from build123d import *

# Parameters (mm, degrees)
SKETCH1_R            = 57
EXTRUDE4_DEPTH       = 7.5
EXTRUDE5_DEPTH       = 7.5
EXTRUDE5_DEPTH_BACK  = 5
SKETCH_R             = 60
SKETCH_R_2           = 57
SKETCH2_R            = 6
SKETCH2_R_2          = 14
EXTRUDE6_DEPTH       = 87.168439698
M5_CLEARANCE_HOLE1_D = 5.5
SKETCH6_R            = 14.8
EXTRUDE7_DEPTH       = 2.5
EXTRUDE8_START       = -16.8000001
EXTRUDE8_OUTLINE_R   = 2
EXTRUDE8_DEPTH       = 2.135757978
EXTRUDE8_START_2     = -3
EXTRUDE8_2_DEPTH     = 6


with BuildPart() as part:
    # Sketch1 → Extrude4 (new, symmetric)
    with BuildSketch(Plane(origin=(0, 0, 0), x_dir=(1, 0, 0), z_dir=(0, 1, 0))):
        with Locations(Location((0, 0, 0), (0, 0, 270))):
            Circle(SKETCH1_R)
    extrude(amount=EXTRUDE4_DEPTH, both=True)

    # Sketch → Extrude5 (add, two sides: drawn at the far end of the back side and taken through both)
    with BuildSketch(Plane(origin=(0, 0, 0), x_dir=(1, 0, 0), z_dir=(0, 1, 0)).offset(-EXTRUDE5_DEPTH_BACK)):
        with Locations(Location((0, 0, 0), (0, 0, 270))):
            Circle(SKETCH_R)
        with Locations(Location((0, 0, 0), (0, 0, 270))):
            Circle(SKETCH_R_2, mode=Mode.SUBTRACT)
    extrude(amount=EXTRUDE5_DEPTH + EXTRUDE5_DEPTH_BACK)

    # Sketch2 → Extrude6 (cut, through all)
    with BuildSketch(Plane(origin=(0, 7.5, 0), x_dir=(1, 0, 0), z_dir=(0, 1, 0))):
        with Locations(Location((-37.5, 0, 0), (0, 0, 270))):
            Circle(SKETCH2_R)
        with Locations(Location((37.5, 0, 0), (0, 0, 270))):
            Circle(SKETCH2_R)
        with Locations(Location((0, 0, 0), (0, 0, 270))):
            Circle(SKETCH2_R_2)
    extrude(amount=-EXTRUDE6_DEPTH, mode=Mode.SUBTRACT)

    # M5 Clearance Hole1 (through all)
    with Locations(Plane(origin=(0, 7.5, 0), x_dir=(1, 0, 0), z_dir=(0, 1, 0))):
        with Locations((37.5, 18), (37.5, -18), (-37.5, 18), (-37.5, -18)):
            Hole(M5_CLEARANCE_HOLE1_D / 2)

    # Sketch6 → Extrude7 (cut, symmetric)
    with BuildSketch(Plane(origin=(0, 0, 0), x_dir=(1, 0, 0), z_dir=(0, 1, 0))):
        with Locations(Location((0, 0, 0), (0, 0, 270))):
            Circle(SKETCH6_R)
    extrude(amount=EXTRUDE7_DEPTH, both=True, mode=Mode.SUBTRACT)

    # Extrude8: read off the stored shape, not the designer's step
    # Extrude8 outline → Extrude8 (cut)
    with BuildSketch(Plane.XY.offset(EXTRUDE8_START)):
        Circle(EXTRUDE8_OUTLINE_R)
    extrude(amount=EXTRUDE8_DEPTH, mode=Mode.SUBTRACT)

    # Extrude8 2 outline → Extrude8 2 (add)
    with BuildSketch(Plane(origin=(0, 0, 0), x_dir=(1, 0, 0), z_dir=(0, 1, 0)).offset(EXTRUDE8_START_2)):
        with BuildLine():
            ThreePointArc((-2e-09, 16.8), (1.002059984, 16.770088723), (2.000551768, 16.680461403))
            Line((2.000551768, 16.680461403), (3, 16.56059374))
            Line((3, 16.56059374), (3, 16.8000001))
            Line((3, 16.8000001), (-2e-09, 16.8))
        make_face()
        with BuildLine():
            ThreePointArc((-2.000001192, 16.680527427), (-1.001783219, 16.770105259), (-2e-09, 16.8))
            Line((-2e-09, 16.8), (-3, 16.8000001))
            Line((-3, 16.8000001), (-3, 16.560627213))
            Line((-3, 16.560627213), (-2.000001192, 16.680527427))
        make_face()
    extrude(amount=EXTRUDE8_2_DEPTH)


solid = part.part
For this review, take the finished solid that the model builds, in its own axes (mm). A direction names the side the tool comes from. Give positions to 0.01 mm unless a question says otherwise; leave off trailing zeros. Loops run counter-clockwise (first coordinate to the right, second up) from the corner with the lowest first, then second, coordinate; pieces in that order, holes last. Notation, with made-up numbers: (34.25, -12.5) -> (89.25, -12.5) arc R19 cw to (89.25, -1.5) -> close; hole circle Ø5 at (12.25, 53). An arc over 180 degrees is marked (long way). One line per question, with ' | ' between items.
1) For faces 4 (the cylindrical face through (40.247, -0.105, 17.879)), 5 (the cylindrical face through (-55.645, -6.232, -12.356)), 6 (the cylindrical face through (-5.67, 0.04, 13.67)), list the 3-axis set-ups (+Z, -Z, +X, -X, +Y, -Y) from which the entire face can be reached by the end or side of a thin tool; tool diameter is ignored.
Resolved:
face 4: +Y, -Y | face 5: -Y | face 6: none
2) The part is to be moulded in two halves that separate along X. For faces 1 (the cylindrical face through (2.64, 1.16, -59.94)), 2 (the flat face through (-11, -2.5, -9)), 3 (the flat face through (-22, -5, 53)), say which applies: +X half, -X half, draft (parallel to the pull), parting line (faces both ways), or undercut.
Resolved:
face 1: parting line | face 2: undercut | face 3: draft
3) We need section B-B (z = 3.5). Write out the cut boundary in (x, y).
Resolved:
outline: (-59.9, -5) -> (-56.89, -5) -> (-56.89, -7.5) -> (-42.37, -7.5) -> (-42.37, 7.5) -> (-59.9, 7.5) -> close; (-32.63, -7.5) -> (-13.56, -7.5) -> (-13.56, -2.5) -> (-14.38, -2.5) -> (-14.38, 2.5) -> (-13.56, 2.5) -> (-13.56, 7.5) -> (-32.63, 7.5) -> close; (13.56, -7.5) -> (32.63, -7.5) -> (32.63, 7.5) -> (13.56, 7.5) -> (13.56, 2.5) -> (14.38, 2.5) -> (14.38, -2.5) -> (13.56, -2.5) -> close; (42.37, -7.5) -> (56.89, -7.5) -> (56.89, -5) -> (59.9, -5) -> (59.9, 7.5) -> (42.37, 7.5) -> close
4) Insertion check: pin 1 Ø7 at (x, z) = (37.5, -18) entering from -Y; pin 2 Ø2 at (y, z) = (1, -36) entering from +X; pin 3 Ø2 at (x, y) = (12.5, 5) entering from +Z; pin 4 Ø6 at (y, z) = (6, -3.5) entering from +X. Each pin has a flat end and moves straight along its axis. Give the tip position at first contact, or say it passes through.
Resolved:
pin 1: stops at y = -7.5 | pin 2: stops at x = 48.73 | pin 3: stops at z = 58.89 | pin 4: stops at x = 60
5) To check wall thickness, follow probe 1 along X at (y, z) = (0.55, 0); probe 2 along X at (y, z) = (-5.5, 0); probe 3 along X at (y, z) = (2, 18). State the ranges of each line that lie inside material, in increasing order.
Resolved:
probe 1: x = -60 to -43.5, -31.5 to -14.8, 14.8 to 31.5, 43.5 to 60 | probe 2: x = -57 to -43.5, -31.5 to -14, 14 to 31.5, 43.5 to 57 | probe 3: x = -57.24 to -40.25, -34.75 to 34.75, 40.25 to 57.24
6) We need section D-D (z = 18). Write out the cut boundary in (x, y), plus the area to 3 significant figures.
Resolved:
outline: (-57.24, -5) -> (-54.08, -5) -> (-54.08, -7.5) -> (-40.25, -7.5) -> (-40.25, 7.5) -> (-57.24, 7.5) -> close; (-34.75, -7.5) -> (34.75, -7.5) -> (34.75, 7.5) -> (-34.75, 7.5) -> close; (40.25, -7.5) -> (54.08, -7.5) -> (54.08, -5) -> (57.24, -5) -> (57.24, 7.5) -> (40.25, 7.5) -> close | area: 1,540 mm2
7) We need section A-A (y = 0). Write out the cut boundary in (x, z), plus the area to 3 significant figures.
Resolved:
outline: circle Ø120 at (0, 0); hole circle Ø12 at (-37.5, 0); hole circle Ø5.5 at (-37.5, -18); hole circle Ø5.5 at (-37.5, 18); hole (-2, -16.68) arc R16.8 ccw to (2, -16.68) -> (2, -14.66) arc R14.8 ccw (long way) to (-2, -14.66) -> close; hole circle Ø12 at (37.5, 0); hole circle Ø5.5 at (37.5, -18); hole circle Ø5.5 at (37.5, 18) | area: 10,300 mm2
8) We need section C-C (x = -8). Write out the cut boundary in (y, z), plus the area to 3 significant figures.
Resolved:
outline: (-7.5, -56.44) -> (-5, -56.44) -> (-5, -59.46) -> (7.5, -59.46) -> (7.5, -11.49) -> (2.5, -11.49) -> (2.5, -12.45) -> (-2.5, -12.45) -> (-2.5, -11.49) -> (-7.5, -11.49) -> close; (-7.5, 11.49) -> (-2.5, 11.49) -> (-2.5, 12.45) -> (2.5, 12.45) -> (2.5, 11.49) -> (7.5, 11.49) -> (7.5, 59.46) -> (-5, 59.46) -> (-5, 56.44) -> (-7.5, 56.44) -> close | area: 1,410 mm2
